For this review, take the finished solid that the model builds, in its own axes (mm). Face numbers are marked on the shaded views. A direction names the side the tool comes from. Round coordinates to 2 decimals unless told otherwise and drop trailing zeros. Loops run counter-clockwise (first coordinate to the right, second up) from the corner with the lowest first, then second, coordinate; pieces in that order, holes last. Notation, with made-up numbers: (-19.75, 83.5) -> (21.25, 83.5) arc R10 cw to (21.25, 89.5) -> close; hole circle Ø8 at (-33, 13). An arc over 180 degrees is marked (long way). Use one line per item in the form item = value. Start each with the question number.
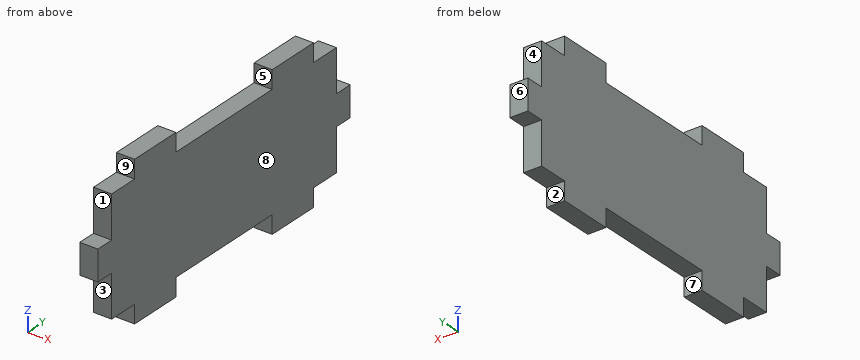
from build123d import *

# Parameters (mm, degrees)
SKETCH_2_W          = 25
SKETCH_2_H          = 55
EXTRUDE_1_DEPTH     = 3
SKETCH_3_W          = 3
SKETCH_3_H          = 8
SKETCH_3_H_2        = 21
CUT_EXTRUDE_1_DEPTH = 4
SKETCH_4_W          = 7
SKETCH_4_H          = 3
CUT_EXTRUDE_2_DEPTH = 4


with BuildPart() as part:
    # 스케치2 → 보스-돌출1 (new body)
    with BuildSketch(Plane(origin=(0, 0, 0), x_dir=(0, 0, -1), z_dir=(1, 0, 0))):
        with Locations((12.5, 27.5)):
            Rectangle(SKETCH_2_W, SKETCH_2_H)
    extrude(amount=EXTRUDE_1_DEPTH)

    # 스케치3 → 컷-돌출1 (cut, through all)
    with BuildSketch(Plane(origin=(3, 0, 0), x_dir=(0, 0, -1), z_dir=(1, 0, 0))):
        with Locations((1.5, 51)):
            Rectangle(SKETCH_3_W, SKETCH_3_H)
        with Locations((23.5, 51)):
            Rectangle(SKETCH_3_W, SKETCH_3_H)
        with Locations((23.5, 27.5)):
            Rectangle(SKETCH_3_W, SKETCH_3_H_2)
        with Locations((1.5, 27.5)):
            Rectangle(SKETCH_3_W, SKETCH_3_H_2)
        with Locations((1.5, 4)):
            Rectangle(SKETCH_3_W, SKETCH_3_H)
        with Locations((23.5, 4)):
            Rectangle(SKETCH_3_W, SKETCH_3_H)
    extrude(amount=-CUT_EXTRUDE_1_DEPTH, mode=Mode.SUBTRACT)

    # 스케치4 → 컷-돌출2 (cut, through all)
    with BuildSketch(Plane(origin=(3, 0, 0), x_dir=(0, 0, -1), z_dir=(1, 0, 0))):
        with Locations((6.5, 53.5)):
            Rectangle(SKETCH_4_W, SKETCH_4_H)
        with Locations((18.5, 53.5)):
            Rectangle(SKETCH_4_W, SKETCH_4_H)
        with Locations((18.5, 1.5)):
            Rectangle(SKETCH_4_W, SKETCH_4_H)
        with Locations((6.5, 1.5)):
            Rectangle(SKETCH_4_W, SKETCH_4_H)
    extrude(amount=-CUT_EXTRUDE_2_DEPTH, mode=Mode.SUBTRACT)


solid = part.part
Item 1: Take a section at A-A on z = -1.5. Give the boundary of the cut face in (x, y).
Item 2: Draft analysis for pull direction Y (two halves, no side actions). For the marked faces 6, 7, 8 and 9, state which applies: +Y half, -Y half, draft (parallel to the pull), parting line (faces both ways), or undercut.
Item 3: Take a section at C-C on y = 33. Give the boundary of the cut face in (x, z), plus the area to 3 significant figures.
Item 4: Take a section at B-B on x = 0.6. Give the boundary of the cut face in (y, z), plus the area to 3 significant figures.
Item 5: Machinability: for the marked faces 1, 2, 3, 4 and 5, which of the approach directions +Z, -Z, +X, -X, +Y, -Y give a long, thin tool a straight path to every point of the face, cutting with its end or side? Answer none if there is none.
Item 6: Wall thickness on line 1 (Y direction, x = 0.5, z = -24); line 2 (Z direction, x = 2.25, y = 7); line 3 (Z direction, x = 1.7, y = 53): over which ranges is each line inside the solid? List them lowest first.
Item 7: Take a section at D-D on z = -18. Give the boundary of the cut face in (x, y).
Item 8: For P1, Ø0.9, axis at x = 2, z = -1, coming from the -Y side; P2, Ø0.9, axis at x = 2, y = 26, coming from the +Z side; P3, Ø1.5, axis at x = 2, z = -1, coming from the +Y side, all flat-tipped, find the tip position at first contact; note any pin that passes through.
Results:
q1.outline = (0, 8) -> (3, 8) -> (3, 17) -> (0, 17) -> close; (0, 38) -> (3, 38) -> (3, 47) -> (0, 47) -> close
q2.face_6 = +Y half
q2.face_7 = undercut
q2.face_8 = draft
q2.face_9 = -Y half
q3.outline = (0, -22) -> (3, -22) -> (3, -3) -> (0, -3) -> close
q3.area = 57.0 mm2
q4.outline = (0, -15) -> (3, -15) -> (3, -22) -> (8, -22) -> (8, -25) -> (17, -25) -> (17, -22) -> (38, -22) -> (38, -25) -> (47, -25) -> (47, -22) -> (52, -22) -> (52, -15) -> (55, -15) -> (55, -10) -> (52, -10) -> (52, -3) -> (47, -3) -> (47, 0) -> (38, 0) -> (38, -3) -> (17, -3) -> (17, 0) -> (8, 0) -> (8, -3) -> (3, -3) -> (3, -10) -> (0, -10) -> close
q4.area = 1,070 mm2
q5.face_1 = +Z, +X, -X, -Y
q5.face_2 = -Z, +X, -X, +Y
q5.face_3 = -Z, +X, -X, -Y
q5.face_4 = +Z, +X, -X, +Y
q5.face_5 = +Z, +X, -X
q6.line_1 = 8 to 17, 38 to 47
q6.line_2 = -22 to -3
q6.line_3 = -15 to -10
q7.outline = (0, 3) -> (3, 3) -> (3, 52) -> (0, 52) -> close
q8.P1 = 8
q8.P2 = -3
q8.P3 = 47
